Can you work these out from the model? Positions are in its coordinate system, mm. Coordinates: 2 decimals unless noted, no trailing zeros. Loops run counter-clockwise (first coordinate to the right, second up) from the corner with the lowest first, then second, coordinate; pieces in that order, holes last.
Autodesk Inventor part; units mm, degrees
ref_plane "YZ Plane" through (0, 0, 0) normal (1, 0, 0) x (0, 1, 0)
ref_plane "XZ Plane" through (0, 0, 0) normal (0, 1, 0) x (-1, 0, 0)
ref_plane "XY Plane" through (0, 0, 0) normal (0, 0, 1) x (1, 0, 0)
sketch "Boceto1" plane through (0, 0, 0) normal (0, 0, 1) x (1, 0, 0)
  line L0 (0, 5) -> (0, 145)
  line L1 (5, 150) -> (30, 150)
  line L2 (35, 145) -> (35, 5)
  line L3 (30, 0) -> (5, 0)
  arc A0 (35, 145) -> (30, 150) centre (30, 145) ccw
  arc A1 (5, 150) -> (0, 145) centre (5, 145) ccw
  arc A2 (0, 5) -> (5, 0) centre (5, 5) ccw
  arc A3 (30, 0) -> (35, 5) centre (30, 5) ccw
  circle A4 centre (17.5, 120) radius 2.5
  circle A5 centre (17.5, 100) radius 2.5
  circle A6 centre (17.5, 80) radius 2.5
  circle A7 centre (17.5, 20) radius 2.5
  point P0 (0, 0)
extrude "Extrusión1" add sketch "Boceto1" along normal blind 3
properties part number "4"
(1) I want a section at B-B on z = 1.15. Write out the boundary of the cut face in (x, y), then the cut area to 3 significant figures.
Check values:
outline: (0, 5) arc R5 ccw to (5, 0) - (30, 0) arc R5 ccw to (35, 5) - (35, 145) arc R5 ccw to (30, 150) - (5, 150) arc R5 ccw to (0, 145) - close; hole circle Ø5 at (17.5, 20); hole circle Ø5 at (17.5, 80); hole circle Ø5 at (17.5, 100); hole circle Ø5 at (17.5, 120)
area: 5,150 mm2
(2) If we mould it in two halves opening along X, with no side actions, what happens to faces 1 (the cylindrical face through (17.17, 97.52, 1.48)), 2 (the cylindrical face through (34, 2, 1)), 3 (the flat face through (18, 0, 1))? For each: released by +X, released by -X, zero draft, split by the parting line, or undercut.
Check values:
face 1: undercut
face 2: released by +X
face 3: zero draft
(3) I want a section at A-A on y = 100. Write out the boundary of the cut face in (x, z), then the cut area to 3 significant figures.
Check values:
outline: (0, 0) - (15, 0) - (15, 3) - (0, 3) - close; (20, 0) - (35, 0) - (35, 3) - (20, 3) - close
area: 90.0 mm2
(4) If I drill on probe 1 along Y at (x, z) = (17.5, 2.15); probe 2 along Y at (x, z) = (30.5, 2.85); probe 3 along X at (y, z) = (102, 2), over which ranges is the centre line in solid material (lowest first)?
Check values:
probe 1: y = 0 to 17.5, 22.5 to 77.5, 82.5 to 97.5, 102.5 to 117.5, 122.5 to 150
probe 2: y = 0.03 to 149.97
probe 3: x = 0 to 16, 19 to 35
